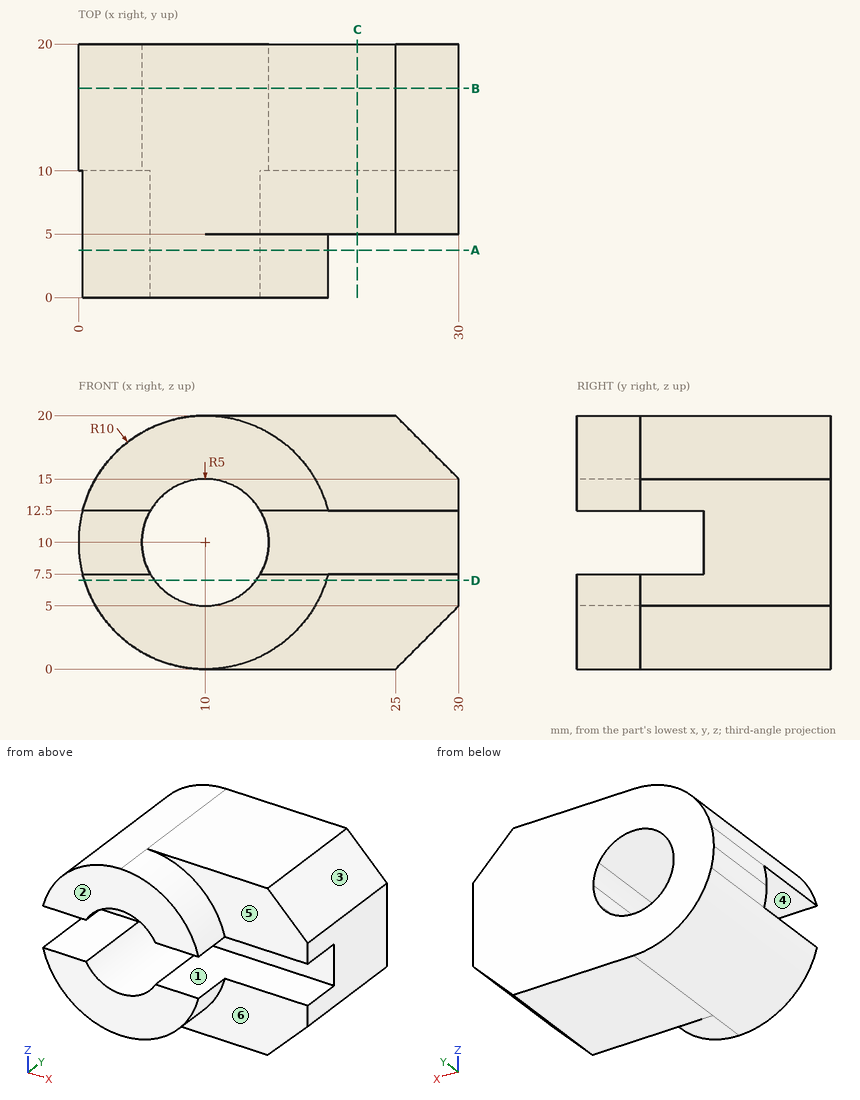
Study the drawing (mm; zero at the part's minimum x, y, z) and answer. A direction names the side the tool comes from. Round coordinates to 2 decimals unless told otherwise and drop trailing zeros. Write each loop counter-clockwise with the first axis right and the second up, starting at its lowest first coordinate (ties: lowest second). Pieces come first, ordered by that corner, then holes. Notation, with made-up numbers: (-16, 51.25) - (-6, 51.25) arc R26 cw to (-6, 90.25) - close; hole circle Ø1 at (87.25, 84.25). An arc over 180 degrees is marked (long way). Return JSON: item names as keys, results as strings. Group by question number.
Q1. For the marked faces 4, 5 and 6, determine the directions among +Z, -Z, +X, -X, +Y, -Y from which every point of the face is accessible in a straight line to the end or side of a thin tool.
Q2. The mould has two halves that part along Z. Classify the marked faces 1, 2 and 3: released by +Z, released by -Z, zero draft, split by the parting line, or undercut.
Q3. The part is cut by section C-C on x = 22. Write down the section's boundary in (y, z), then the cut area to 3 significant figures.
Q4. The part is cut by section A-A on y = 3.75. Write down the section's boundary in (x, z).
Q5. Find the intervals of material crossed by L1, parallel to Y at x = 26.5, z = 7.25; L2, parallel to Z at x = 4, y = 7; L3, parallel to Y at x = 4, z = 7.75, in increasing order.
Q6. The part is cut by section D-D on z = 7. Write down the section's boundary in (x, y).
Q7. The part is cut by section B-B on y = 16.5. Write down the section's boundary in (x, z).
Q8. Each of these flat-tipped pins is pushed along its axis until it touches: pin 1 Ø1.5 at (x, z) = (19, 10.5) entering from -Y; pin 2 Ø8 at (x, y) = (12.5, 3.5) entering from +Z; pin 3 Ø2.5 at (x, y) = (3, 5) entering from -Z; pin 4 Ø2.5 at (x, z) = (19.5, 2) entering from -Y. Where does it stop, or does it pass through?
Solved:
{
 "1": {"face 4": "+X, -X, -Y", "face 5": "+Z, +X, -Y", "face 6": "-Z, +X, -Y"},
 "2": {"face 1": "undercut", "face 2": "zero draft", "face 3": "released by +Z"},
 "3": {"outline": "(5, 0) - (20, 0) - (20, 20) - (5, 20) - (5, 12.5) - (10, 12.5) - (10, 7.5) - (5, 7.5) - close", "area": "275 mm²"},
 "4": {"outline": "(0.32, 7.5) arc R10 ccw to (19.68, 7.5) - (14.33, 7.5) arc R5 cw to (5.67, 7.5) - close; (0.32, 12.5) - (5.67, 12.5) arc R5 cw to (14.33, 12.5) - (19.68, 12.5) arc R10 ccw to start"},
 "5": {"L1": "5 to 20", "L2": "2 to 7.5, 12.5 to 18", "L3": "10 to 20"},
 "6": {"outline": "(0.46, 0) - (6, 0) - (6, 20) - (0.46, 20) - close; (14, 0) - (19.54, 0) - (19.54, 5) - (30, 5) - (30, 20) - (14, 20) - close"},
 "7": {"outline": "(10, 0) - (25, 0) - (30, 5) - (30, 15) - (25, 20) - (10, 20) arc R10 ccw to start; hole circle Ø10 at (10, 10)"},
 "8": {"pin 1": "y = 10", "pin 2": "z = 20", "pin 3": "z = 1.82", "pin 4": "y = 5"}
}
